Source: CAD feature listing. Evaluate the final solid. Frame: model axes, mm. Face numbers are marked on the shaded views. Give positions to 0.01 mm unless a question says otherwise; leave off trailing zeros. Loops run counter-clockwise (first coordinate to the right, second up) from the corner with the lowest first, then second, coordinate; pieces in that order, holes last. Notation, with made-up numbers: M -35,9 L -1,9 A14 ccw -1,35 Z; hole C 12,-7 d4. An arc over 180 degrees is marked long. Put each result on its own line as item: value.
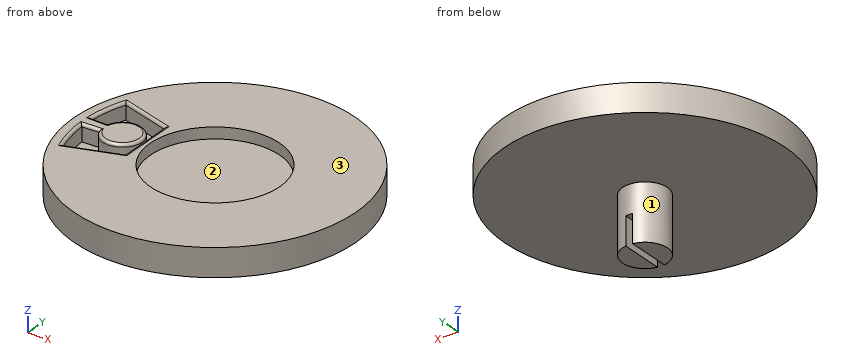
from build123d import *

# Parameters (mm, degrees)
SKETCH1_R           = 25
BOSS_EXTRUDE1_DEPTH = 5
CUT_EXTRUDE1_START  = 5
CUT_EXTRUDE1_DEPTH  = 3
CUT_EXTRUDE2_START  = 5
SKETCH3_R           = 11.5
CUT_EXTRUDE2_DEPTH  = 2
SKETCH4_R           = 4
BOSS_EXTRUDE2_DEPTH = 10
CUT_EXTRUDE3_START  = -10
SKETCH5_W           = 1.2
SKETCH5_H           = 10
CUT_EXTRUDE3_DEPTH  = 5
FILLET1_R           = 0.5


with BuildPart() as part:
    # Sketch1 → Boss-Extrude1 (new body)
    with BuildSketch(Plane.XY):
        Circle(SKETCH1_R)
    extrude(amount=BOSS_EXTRUDE1_DEPTH)

    # Sketch2 → Cut-Extrude1 (cut)
    with BuildSketch(Plane.XY.offset(CUT_EXTRUDE1_START)):
        with BuildLine():
            Line((-19.920587104, -1.094962553), (-22.96853355, -1.202691377))
            ThreePointArc((-22.96853355, -1.202691377), (-22.537445492, -4.589504406), (-21.609752304, -7.875189228))
            Line((-21.609752304, -7.875189228), (-12.555769306, -4.868581062))
            Line((-12.555769306, -4.868581062), (-12.669871245, 5.133277845))
            Line((-12.669871245, 5.133277845), (-21.609327517, 7.876354758))
            ThreePointArc((-21.609327517, 7.876354758), (-22.540397078, 4.574986289), (-22.970127121, 1.171861786))
            Line((-22.970127121, 1.171861786), (-19.990271583, 1.051061802))
            ThreePointArc((-19.990271583, 1.051061802), (-13.12774726, 0.199754222), (-19.920587104, -1.094962553))
        make_face()
    extrude(amount=-CUT_EXTRUDE1_DEPTH, mode=Mode.SUBTRACT)

    # Sketch3 → Cut-Extrude2 (cut)
    with BuildSketch(Plane.XY.offset(CUT_EXTRUDE2_START)):
        Circle(SKETCH3_R)
    extrude(amount=-CUT_EXTRUDE2_DEPTH, mode=Mode.SUBTRACT)

    # Sketch4 → Boss-Extrude2 (add)
    with BuildSketch(Plane.XY):
        Circle(SKETCH4_R)
    extrude(amount=-BOSS_EXTRUDE2_DEPTH)

    # Sketch5 → Cut-Extrude3 (cut)
    with BuildSketch(Plane.XY.offset(CUT_EXTRUDE3_START)):
        Rectangle(SKETCH5_W, SKETCH5_H)
    extrude(amount=CUT_EXTRUDE3_DEPTH, mode=Mode.SUBTRACT)

    # Fillet1
    fillet1_edges = [part.edges().sort_by_distance(p)[0] for p in [
        (-17.082760805, -6.371885145, 5),
        (-21.444560327, -1.148826965, 5),
        (-13.12774726, 0.199754222, 5),
        (-21.480199352, 1.111461794, 5),
        (-22.540397078, 4.574986289, 5),
        (-22.537445492, -4.589504406, 5),
        (-17.139599381, 6.504816302, 5),
        (-12.612820275, 0.132348391, 5),
    ]]
    fillet(fillet1_edges, radius=FILLET1_R)


solid = part.part
1. Draft query along Y for the marked faces 1, 2 and 3. Return one class per face: pulls with the +Y half, pulls with the -Y half, needs draft (parallel to the pull), parting line crosses it, or undercut.
Found:
face 1: parting line crosses it
face 2: undercut
face 3: needs draft
2. Contact query for flat-ended pins moving along their axis: P1, Ø4, axis at x = 18, y = 20, coming from the -Z side; P2, Ø6, axis at x = -8, z = -8, coming from the +Y side; P3, Ø4, axis at y = 0.5, z = -7.5, coming from the +X side; P4, Ø1.5, axis at y = 0, z = -6.5, coming from the -X side. Output: stop coordinate, or through.
Found:
P1: z = 0
P2: through
P3: x = 4
P4: x = -4
3. Section query D-D (y = 15). Output: boundary loops of the cut face in (x, z).
Found:
outline: M -20,0 L 20,0 L 20,5 L -20,5 Z
4. Section query B-B (x = 0). Output: boundary loops of the cut face in (y, z).
Found:
outline: M -25,0 L -4,0 L -4,-5 L 4,-5 L 4,0 L 25,0 L 25,5 L 11.5,5 L 11.5,3 L -11.5,3 L -11.5,5 L -25,5 Z
5. Material intervals for line 1 (Y direction, x = 0, z = 3.6); line 2 (Z direction, x = -1, y = -3.5); line 3 (Z direction, x = -17.5, y = 12.5), sorted ascending. Write a range as from..to.
Found:
line 1: -25..-11.5, 11.5..25
line 2: -10..3
line 3: 0..5
6. Section query A-A (z = -7.75). Output: boundary loops of the cut face in (x, y).
Found:
outline: M -0.6,-3.95 L -0.6,3.95 A4 ccw Z; M 0.6,-3.95 A4 ccw 0.6,3.95 Z
7. Section query C-C (z = 0.75). Output: boundary loops of the cut face in (x, y).
Found:
outline: C 0,0 d50
